Input: part model. Units: mm. Frame: model coordinates. Coordinates: 2 decimals unless noted, no trailing zeros. Order: outer loops, then holes, each group sorted by start corner. A loop starts at its lowest first (then second) coordinate and runs counter-clockwise, first axis right, second up.
from build123d import *

# Parameters (mm, degrees)
SKETCH_1_W                   = 545
SKETCH_1_H                   = 12
EXTRUDE_1_DEPTH              = 8
CUT_EXTRUDE_1_DEPTH          = 546.047704334
CUT_EXTRUDE_2_DEPTH          = 546.047704334
CUT_EXTRUDE_3_DEPTH          = 546.047704334
CUT_EXTRUDE_4_DEPTH          = 546.047704334
CUT_EXTRUDE_5_DEPTH          = 546.047704334
CUT_EXTRUDE_6_DEPTH          = 546.047704334
HOLE_WIZARD_M3_1_D           = 3.5
HOLE_WIZARD_M3_1_CBORE_D     = 5.9999
HOLE_WIZARD_M3_1_CBORE_DEPTH = 4.5
CHAMFER_1_SIZE               = 0.6
FILLET_1_R                   = 0.2


with BuildPart() as part:
    # 草图1 → 凸台-拉伸1 (new body)
    with BuildSketch(Plane(origin=(0, 4, 0), x_dir=(1, 0, 0), z_dir=(0, 1, 0))):
        Rectangle(SKETCH_1_W, SKETCH_1_H)
    extrude(amount=-EXTRUDE_1_DEPTH)

    # 草图2 → 切除-拉伸1 (cut, through all)
    with BuildSketch(Plane(origin=(272.5, 0, 0), x_dir=(0, 0, -1), z_dir=(1, 0, 0))):
        with BuildLine():
            Line((6, 1.51), (6, 2.01))
            Line((6, 2.01), (4.8, 2.01))
            ThreePointArc((4.8, 2.01), (4.55, 1.76), (4.8, 1.51))
            Line((4.8, 1.51), (6, 1.51))
        make_face()
    extrude(amount=-CUT_EXTRUDE_1_DEPTH, mode=Mode.SUBTRACT)

    # 草图3 → 切除-拉伸2 (cut, through all)
    with BuildSketch(Plane(origin=(272.5, 0, 0), x_dir=(0, 0, -1), z_dir=(1, 0, 0))):
        with BuildLine():
            Line((6, 2.01), (6, 3.111111))
            ThreePointArc((6, 3.111111), (5.367595703, 2.693428684), (5.04, 2.01))
            Line((5.04, 2.01), (6, 2.01))
        make_face()
    extrude(amount=-CUT_EXTRUDE_2_DEPTH, mode=Mode.SUBTRACT)

    # 草图4 → 切除-拉伸3 (cut, through all)
    with BuildSketch(Plane(origin=(272.5, 0, 0), x_dir=(0, 0, -1), z_dir=(1, 0, 0))):
        with BuildLine():
            Line((6, 1.51), (5.04, 1.51))
            ThreePointArc((5.04, 1.51), (5.367595703, 0.826571316), (6, 0.408889))
            Line((6, 0.408889), (6, 1.51))
        make_face()
    extrude(amount=-CUT_EXTRUDE_3_DEPTH, mode=Mode.SUBTRACT)

    # 草图5 → 切除-拉伸4 (cut, through all)
    with BuildSketch(Plane(origin=(272.5, 0, 0), x_dir=(0, 0, -1), z_dir=(1, 0, 0))):
        with BuildLine():
            Line((-6, 2.01), (-6, 1.51))
            Line((-6, 1.51), (-4.8, 1.51))
            ThreePointArc((-4.8, 1.51), (-4.55, 1.76), (-4.8, 2.01))
            Line((-4.8, 2.01), (-6, 2.01))
        make_face()
    extrude(amount=-CUT_EXTRUDE_4_DEPTH, mode=Mode.SUBTRACT)

    # 草图6 → 切除-拉伸5 (cut, through all)
    with BuildSketch(Plane(origin=(272.5, 0, 0), x_dir=(0, 0, -1), z_dir=(1, 0, 0))):
        with BuildLine():
            Line((-6, 1.51), (-6, 0.408889))
            ThreePointArc((-6, 0.408889), (-5.367595703, 0.826571316), (-5.04, 1.51))
            Line((-5.04, 1.51), (-6, 1.51))
        make_face()
    extrude(amount=-CUT_EXTRUDE_5_DEPTH, mode=Mode.SUBTRACT)

    # 草图7 → 切除-拉伸6 (cut, through all)
    with BuildSketch(Plane(origin=(272.5, 0, 0), x_dir=(0, 0, -1), z_dir=(1, 0, 0))):
        with BuildLine():
            Line((-6, 2.01), (-5.04, 2.01))
            ThreePointArc((-5.04, 2.01), (-5.367595703, 2.693428684), (-6, 3.111111))
            Line((-6, 3.111111), (-6, 2.01))
        make_face()
    extrude(amount=-CUT_EXTRUDE_6_DEPTH, mode=Mode.SUBTRACT)

    # M3 六角头机械螺钉的柱形沉头孔1 (through all)
    with Locations(Plane(origin=(0, 4, 0), x_dir=(1, 0, 0), z_dir=(0, 1, 0))):
        with Locations((-262.5, 0), (-237.5, 0), (-212.5, 0), (-187.5, 0), (-162.5, 0), (-137.5, 0), (-112.5, 0), (-87.5, 0), (-62.5, 0), (-37.5, 0), (-12.5, 0), (12.5, 0), (37.5, 0), (62.5, 0), (87.5, 0), (112.5, 0), (137.5, 0), (162.5, 0), (187.5, 0), (212.5, 0), (237.5, 0), (262.5, 0)):
            CounterBoreHole(HOLE_WIZARD_M3_1_D / 2, HOLE_WIZARD_M3_1_CBORE_D / 2, HOLE_WIZARD_M3_1_CBORE_DEPTH)

    # 倒角1
    chamfer_1_edges = [part.edges().sort_by_distance(p)[0] for p in [
        (0, -4, -6),
        (0, -4, 6),
    ]]
    chamfer(chamfer_1_edges, length=CHAMFER_1_SIZE)

    # 圆角1
    fillet_1_edges = [part.edges().sort_by_distance(p)[0] for p in [
        (0, 2.01, -5.04),
        (0, 3.111111, -6),
        (0, 0.408889, -6),
        (0, 1.51, -5.04),
        (0, 4, -6),
        (0, 4, 6),
        (0, 1.51, 5.04),
        (0, 0.408889, 6),
        (0, 3.111111, 6),
        (0, 2.01, 5.04),
    ]]
    fillet(fillet_1_edges, radius=FILLET_1_R)


solid = part.part
Item 1: Pin query (flat end, axial travel): pin 1 Ø1.8 at (x, z) = (-86.5, 1) entering from +Y. Return the tip coordinate at first contact, or that it passes through.
Response values:
pin 1: stops at y = -0.5
Item 2: Ray query, probe 1 along Y at (x, z) = (-39.5, 5); probe 2 along Z at (x, y) = (-215, 1.75); probe 3 along Z at (x, y) = (137.5, 3.05). Return the intervals inside material, ascending.
Response values:
probe 1: y = -4 to 1.47, 2.05 to 4
probe 2: z = -4.55 to -1.66, 1.66 to 4.55
probe 3: z = -5.84 to -3, 3 to 5.84
Item 3: Cut plane A-A on x = -97.5. Return loops of the section in (y, z), then the cut area to 3 significant figures.
Response values:
outline: (-4, -5.4) - (-3.4, -6) - (0.27, -6) arc R0.2 ccw to (0.45, -5.88) arc R1.42 cw to (1.37, -5.07) arc R0.2 ccw to (1.51, -4.88) - (1.51, -4.8) arc R0.25 cw to (2.01, -4.8) - (2.01, -4.88) arc R0.2 ccw to (2.15, -5.07) arc R1.42 cw to (3.07, -5.88) arc R0.2 ccw to (3.25, -6) - (3.8, -6) arc R0.2 ccw to (4, -5.8) - (4, 5.8) arc R0.2 ccw to (3.8, 6) - (3.25, 6) arc R0.2 ccw to (3.07, 5.88) arc R1.42 cw to (2.15, 5.07) arc R0.2 ccw to (2.01, 4.88) - (2.01, 4.8) arc R0.25 cw to (1.51, 4.8) - (1.51, 4.88) arc R0.2 ccw to (1.37, 5.07) arc R1.42 cw to (0.45, 5.88) arc R0.2 ccw to (0.27, 6) - (-3.4, 6) - (-4, 5.4) - close
area: 91.3 mm2
